Could you check a few things on this model? Use its own coordinates, in mm. Give positions to 0.01 mm unless a question says otherwise; leave off trailing zeros. Order: outer loops, then holes, each group sorted by start corner. A loop starts at its lowest first (then second) coordinate and runs counter-clockwise, first axis right, second up. Notation, with made-up numbers: (77.25, -40) - (90.25, -40) arc R17 ccw to (90.25, -32) - close; hole circle Ø5 at (74, 85). An arc over 180 degrees is marked (long way). Put each result on its own line as item: value.
Autodesk Inventor part; units mm, degrees
ref_plane "YZ Plane" through (0, 0, 0) normal (1, 0, 0) x (0, 1, 0)
ref_plane "XZ Plane" through (0, 0, 0) normal (0, 1, 0) x (-1, 0, 0)
ref_plane "XY Plane" through (0, 0, 0) normal (0, 0, 1) x (1, 0, 0)
sketch "Sketch1" plane through (0, 0, 0) normal (0, 0, 1) x (1, 0, 0)
  line L0 (-25, 25) -> (25, 25)
  line L1 (25, 25) -> (25, -25)
  line L2 (25, -25) -> (-25, -25)
  line L3 (-25, -25) -> (-25, 25)
  line L4 (22.5, 22.5) -> (-22.5, 22.5)
  line L5 (-22.5, 22.5) -> (-22.5, -22.5)
  line L6 (-22.5, -22.5) -> (22.5, -22.5)
  line L7 (22.5, -22.5) -> (22.5, 22.5)
  point P0 (0, 0)
  dimension "d0" = 50
  dimension "d1" = 50
  dimension "d2" = 25
  dimension "d3" = 25
  dimension "d4" = 2.5
extrude "Extrusion1" add sketch "Sketch1" along normal blind 990
fillet "Fillet1" radius 2 4 edges at (25, 25, 495) (-25, 25, 495) (25, -25, 495) (-25, -25, 495)
sketch "Sketch2" plane through (-23, 25, 0) normal (0, 1, 0) x (1, 0, 0)
  line L0 (46, 0) -> (0, 0)
  line L1 (46, -990) -> (0, -990)
  point P0 (23, 0)
  point P1 (23, -45)
  point P2 (23, -945)
  dimension "d8" = 45
  dimension "d9" = 0
  dimension "d10" = 45
  dimension "d11" = 0
hole "endHoles" at (0, 25, 45) at (0, 25, 945) direction (0, -1, 0) diameter 10 depth 2.5
sketch "Sketch3" plane through (25, -23, 0) normal (1, 0, 0) x (0, 0, -1)
  point P0 (0, 23)
  point P1 (-860, 23)
  point P2 (-760, 23)
  dimension "d19" = 860
  dimension "d20" = 760
  dimension "d21" = 0
  dimension "d22" = 0
hole "clampHoles" at (25, 0, 860) at (25, 0, 760) direction (-1, 0, 0) diameter 10 end through all
sketch "Sketch4" plane through (-25, -23, 0) normal (-1, 0, 0) x (0, 0, 1)
  circle A0 centre (760, 23) radius 5
  circle A1 centre (760, 23) radius 5
  circle A2 centre (860, 23) radius 5
  line L0 (760, 23) -> (860, 23)
  point P0 (0, 23)
  point P1 (790.4, 23)
  point P2 (820.4, 23)
  dimension "d30" = 30
  dimension "d32" = 39.6
hole "Hole3" at (-25, 0, 790.4) at (-25, 0, 820.4) direction (1, 0, 0) diameter 10 end through all
equation "\"d0\" = w"
equation "\"d1\" = w"
equation "\"d4\" = 0.5 * t"
equation "\"d5\" = L + 2 * buffer"
equation "\"d7\" = fillet"
equation "\"d23\" = support_frame_clampHoleDiameter"
equation "\"w\" = support_frame_squareBarDimension"
equation "\"t\" = support_frame_squareBarThickness"
equation "\"fillet\" = support_frame_squareBarFillet"
equation "\"support_frame_endHoleBuffer\" = 45"
equation "\"buffer\" = support_frame_endHoleBuffer"
equation "\"hoop_angle_z\" = 45deg"
equation "\"hoop_bearing_length\" = 5deg"
equation "\"hoop_cable_diam\" = 5"
equation "\"hoop_cable_pulley_diam\" = 22"
equation "\"hoop_thickness_large\" = 4"
equation "\"hoop_thickness_medium\" = 3.2"
equation "\"hoop_thickness_small\" = 2"
equation "\"hoop_width_large\" = 51"
equation "\"hoop_width_medium\" = 33.7"
equation "\"hoop_width_small\" = 25.4"
equation "\"rack_tooth_addendum\" = 5"
equation "\"rack_tooth_dedendum\" = 5"
equation "\"rack_tooth_thickness\" = 5"
equation "\"secure_arm_angle\" = 35deg"
equation "\"secure_arm_radii\" = 9"
equation "\"support_baseClamp_platformLengthBuffer\" = 35"
equation "\"support_baseClamp_platformThickness\" = 15"
equation "\"support_baseClamp_platformWidthBuffer\" = 0"
equation "\"support_baseClamp_sleeveHoleDiameter\" = 12"
equation "\"support_baseClamp_sleeveSweepTerminationAngle\" = 55deg"
equation "\"support_baseClamp_thickness\" = 8"
equation "\"support_frame_clampHoleDiameter\" = 10"
equation "\"support_frame_squareBarFillet\" = 2"
equation "\"support_frame_squareBarThickness\" = 5"
equation "\"hoop_tabs_thickness\" = 6"
equation "\"wheelchair_deployed_length\" = 1067"
equation "\"wheelchair_deployed_height\" = 914"
equation "\"hoop_tabs_hole\" = 12"
equation "\"wheelchair_deployed_width\" = 635"
equation "\"sm_varx_pinPlate_thickness\" = 5"
equation "\"sm_varx_member_tolerance\" = 0"
equation "\"sm_varx_pinPlate_holeDiameter\" = 5"
equation "\"sm_varx_squareBarThickness\" = 2.5"
equation "\"hoop_bushing23_radialInterference\" = 0"
equation "\"hoop_bushing12_radialInterference\" = 0"
equation "\"hoop_bushing12_od\" = -2 * hoop_thickness_large + hoop_width_large + hoop_bushing12_radialInterference"
equation "\"wheelchatir_pos_deploy_angle_0\" = 65deg"
equation "\"wheelchatir_pos_store_angle_0\" = 90deg"
equation "\"wheelchatir_pos_deploy_angle_1\" = 20deg"
equation "\"wheelchatir_pos_store_angle_1\" = 20deg"
equation "\"hoop_bushing23_od\" = -2 * hoop_thickness_medium + hoop_width_medium + hoop_bushing23_radialInterference"
equation "\"hoop_bushing12_thickness\" = -hoop_width_medium + hoop_bushing12_od - 2 * hoop_bushing12_radialInterference"
equation "\"hoop_bushing23_thickness\" = -hoop_width_small + hoop_bushing23_od - 2 * hoop_bushing23_radialInterference"
properties part number "support_frame_x" material "Steel, Mild"
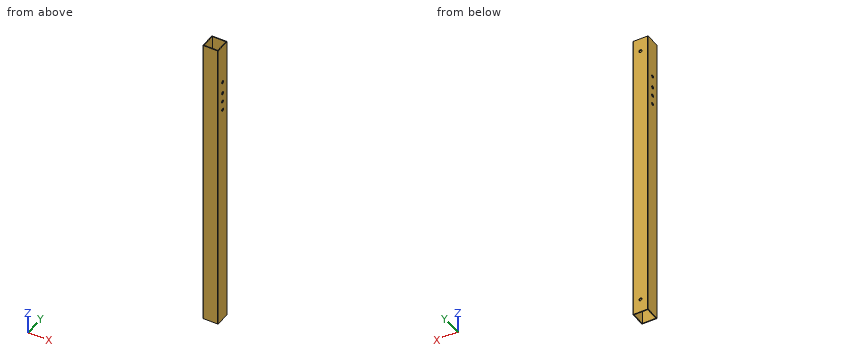
1) Suppose I cut it at A-A, the plane x = 15. List the corners of the cut face in (y, z) for me.
Filled in:
outline: (-25, 0) - (-22.5, 0) - (-22.5, 990) - (-25, 990) - close; (22.5, 0) - (25, 0) - (25, 990) - (22.5, 990) - close
2) If I drill on line 1 (Z direction, x = -23.1, y = 0); line 2 (Y direction, x = -8, z = 119), over which ranges is the centre line in solid material (lowest first)? Write a range as [from, to].
Filled in:
line 1: z = [0, 755], [765, 785.4], [795.4, 815.4], [825.4, 855], [865, 990]
line 2: y = [-25, -22.5], [22.5, 25]
3) Suppose I cut it at C-C, the plane z = 128.5. List the corners of the cut face in (x, y) for me, and give its area (3 significant figures).
Filled in:
outline: (-25, -23) arc R2 ccw to (-23, -25) - (23, -25) arc R2 ccw to (25, -23) - (25, 23) arc R2 ccw to (23, 25) - (-23, 25) arc R2 ccw to (-25, 23) - close; hole (-22.5, -22.5) - (22.5, -22.5) - (22.5, 22.5) - (-22.5, 22.5) - close
area: 472 mm^2
4) I'm going to push a flat-ended pin straight in: pin 1 (9 mm diameter, centred on y = 0, z = 820.4, fed in from +X). Where does the tip first touch, or does it pass through?
Filled in:
pin 1: passes through
